Geometry check sheet. Reference: the model listing, model coordinates, mm. Face numbers are marked on the shaded views. A direction names the side the tool comes from. Coordinates: 2 decimals unless noted, no trailing zeros. Order: outer loops, then holes, each group sorted by start corner. A loop starts at its lowest first (then second) coordinate and runs counter-clockwise, first axis right, second up. Notation, with made-up numbers: (23.5, 75) -> (31.5, 75) arc R19 cw to (31.5, 98) -> close; hole circle Ø1 at (43.25, 61). An arc over 180 degrees is marked (long way). Answer in a Markdown table with one row per item. Add a question column.
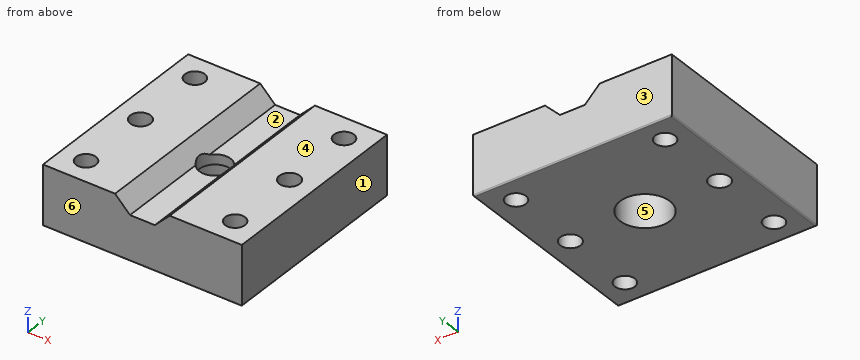
```python
from build123d import *

# Parameters (mm, degrees)
F0_W      = 40
F0_H      = 40
F1_DEPTH  = 12
F3_DEPTH  = 40.001
F4_R      = 2
F5_DEPTH  = 12.001
F6_R      = 2.05
F7_DEPTH  = 12.001
F8_R      = 0.25
F9_R      = 3.15
F10_DEPTH = 12.001
F11_R     = 5
F12_DEPTH = 7


with BuildPart() as f1:
    # F0 (on Top) → F1 (new body)
    with BuildSketch(Plane.XY):
        with Locations((20, 20)):
            Rectangle(F0_W, F0_H)
    extrude(amount=F1_DEPTH)

    # F2 (on face) → F3 (cut, through all)
    with BuildSketch(Plane.XZ):
        Polygon((14.5, 12), (17.5, 9), (22.5, 9), (25.5, 12), align=None)
    extrude(amount=-F3_DEPTH, mode=Mode.SUBTRACT)

    # F4 (on face) → F5 (cut, through all)
    with BuildSketch(Plane.XY.offset(12)):
        with Locations((5, 5)):
            Circle(F4_R)
        with Locations((5, 35)):
            Circle(F4_R)
        with Locations((35, 5)):
            Circle(F4_R)
        with Locations((35, 35)):
            Circle(F4_R)
    extrude(amount=-F5_DEPTH, mode=Mode.SUBTRACT)

    # F6 (on face) → F7 (cut, through all)
    with BuildSketch(Plane.XY.offset(12)):
        with Locations((5, 20)):
            Circle(F6_R)
        with Locations((35, 20)):
            Circle(F6_R)
    extrude(amount=-F7_DEPTH, mode=Mode.SUBTRACT)

    # F8
    f8_edges = [f1.edges().sort_by_distance(p)[0] for p in [
        (20, 0, 0),
        (0, 20, 0),
        (40, 20, 0),
        (20, 40, 0),
    ]]
    fillet(f8_edges, radius=F8_R)

    # F9 (on face) → F10 (cut, through all)
    with BuildSketch(Plane(origin=(0, 0, 0), x_dir=(1, 0, 0), z_dir=(0, 0, -1))):
        with Locations((20, -20)):
            Circle(F9_R)
    extrude(amount=-F10_DEPTH, mode=Mode.SUBTRACT)

    # F11 (on face) → F12 (cut)
    with BuildSketch(Plane(origin=(0, 0, 0), x_dir=(1, 0, 0), z_dir=(0, 0, -1))):
        with Locations((20, -20)):
            Circle(F11_R)
    extrude(amount=-F12_DEPTH, mode=Mode.SUBTRACT)


solid = f1.part
```
(1) Cross-section at B-B (z = 4.5). Enter the section's corners in (x, y).
(2) Cross-section at C-C (x = 20). Enter the section's corners in (y, z).
(3) Cross-section at A-A (y = 5). Enter the section's corners in (x, z).
(4) Cross-section at D-D (x = 35). Enter the section's corners in (y, z), plus the area to 3 significant figures.
(5) Mould release check, pull along Y, two halves, no side actions. Record for the marked faces 3, 4, 5 and 6: +Y half, -Y half, draft (parallel to the pull), parting line (faces both ways), or undercut.
(6) Scan lines: line 1 along Y through (x, z) = (5, 4.5); line 2 along X through (y, z) = (6, 10.5); line 3 along Y through (x, z) = (5.5, 7). Record each from-to range of solid material in increasing order.
(7) Go/stop test with flat-tipped pins: P1, Ø1.5, axis at x = 20.5, y = 11, coming from the +Z side; P2, Ø3, axis at x = 20, y = 17.5, coming from the -Z side. Record where each tip stops, or that it passes through.
(8) Access from +Z, -Z, +X, -X, +Y, -Y to the whole of each face (thin tool, end or side, straight path). Record for the marked faces 1 and 2.
Checks:
| question | item | result |
|---|---|---|
| 1 | outline | (0, 0) -> (40, 0) -> (40, 40) -> (0, 40) -> close; hole circle Ø4.1 at (5, 20); hole circle Ø4 at (5, 5); hole circle Ø4 at (5, 35); hole circle Ø10 at (20, 20); hole circle Ø4.1 at (35, 20); hole circle Ø4 at (35, 5); hole circle Ø4 at (35, 35) |
| 2 | outline | (0, 0.25) arc R0.25 ccw to (0.25, 0) -> (15, 0) -> (15, 7) -> (16.85, 7) -> (16.85, 9) -> (0, 9) -> close; (23.15, 7) -> (25, 7) -> (25, 0) -> (39.75, 0) arc R0.25 ccw to (40, 0.25) -> (40, 9) -> (23.15, 9) -> close |
| 3 | outline | (0, 0.25) arc R0.25 ccw to (0.25, 0) -> (3, 0) -> (3, 12) -> (0, 12) -> close; (7, 0) -> (33, 0) -> (33, 12) -> (25.5, 12) -> (22.5, 9) -> (17.5, 9) -> (14.5, 12) -> (7, 12) -> close; (37, 0) -> (39.75, 0) arc R0.25 ccw to (40, 0.25) -> (40, 12) -> (37, 12) -> close |
| 4 | outline | (0, 0.25) arc R0.25 ccw to (0.25, 0) -> (3, 0) -> (3, 12) -> (0, 12) -> close; (7, 0) -> (17.95, 0) -> (17.95, 12) -> (7, 12) -> close; (22.05, 0) -> (33, 0) -> (33, 12) -> (22.05, 12) -> close; (37, 0) -> (39.75, 0) arc R0.25 ccw to (40, 0.25) -> (40, 12) -> (37, 12) -> close |
| 4 | area | 335 mm² |
| 5 | face 3 | +Y half |
| 5 | face 4 | draft |
| 5 | face 5 | undercut |
| 5 | face 6 | -Y half |
| 6 | line 1 | 0 to 3, 7 to 17.95, 22.05 to 33, 37 to 40 |
| 6 | line 2 | 0 to 3.27, 6.73 to 16, 24 to 33.27, 36.73 to 40 |
| 6 | line 3 | 0 to 3.06, 6.94 to 18.01, 21.99 to 33.06, 36.94 to 40 |
| 7 | P1 | z = 9 |
| 7 | P2 | z = 7 |
| 8 | face 1 | +Z, -Z, +X, +Y, -Y |
| 8 | face 2 | +Z, +Y, -Y |
